```python
from build123d import *

# Parameters (mm, degrees)
SKETCH2_R           = 1.3
CUT_EXTRUDE1_DEPTH  = 15
BOSS_EXTRUDE1_START = 6
SKETCH3_R           = 2
SKETCH3_R_2         = 1.3
BOSS_EXTRUDE1_DEPTH = 6


with BuildPart() as part:
    # Sketch1 → Revolve2 (revolve)
    with BuildSketch(Plane.XY):
        with BuildLine():
            Line((-2.5, 0), (2.5, 0))
            ThreePointArc((2.5, 0), (0, -2.5), (-2.5, 0))
        make_face()
    revolve(axis=Axis((4.664316952, 0, 0), (-1, 0, 0)))

    # Sketch2 → Cut-Extrude1 (cut, symmetric)
    with BuildSketch(Plane(origin=(0, 0, 0), x_dir=(1, 0, 0), z_dir=(0, 1, 0))):
        with Locations(Location((0, 0, 0), (0, 0, 90))):
            Circle(SKETCH2_R)
    extrude(amount=CUT_EXTRUDE1_DEPTH, both=True, mode=Mode.SUBTRACT)

    # Sketch3 → Boss-Extrude1 (add)
    with BuildSketch(Plane(origin=(0, 0, 0), x_dir=(1, 0, 0), z_dir=(0, 1, 0)).offset(BOSS_EXTRUDE1_START)):
        with Locations(Location((0, 0, 0), (0, 0, 270))):
            Circle(SKETCH3_R)
        with Locations(Location((0, 0, 0), (0, 0, 270))):
            Circle(SKETCH3_R_2, mode=Mode.SUBTRACT)
    extrude(amount=-BOSS_EXTRUDE1_DEPTH)


solid = part.part
```
Could you check a few things on this model? Use its own coordinates, in mm. Coordinates: 2 decimals unless noted, no trailing zeros. Order: outer loops, then holes, each group sorted by start corner. A loop starts at its lowest first (then second) coordinate and runs counter-clockwise, first axis right, second up. Notation, with made-up numbers: M 1,78 L 21,78 A25 ccw 21,107 Z; hole C 77,-6 d7. An arc over 180 degrees is marked long. Use a Markdown table: item, result. Add a question column.
Q1. I want a section at C-C on y = 3.25. List the corners of the cut face in (x, z) for me.
Q2. I want a section at D-D on y = 1.25. List the corners of the cut face in (x, z) for me, then the cut area to 3 significant figures.
Q3. I'm going to push flat-ended pins straight in: pin 1 (1 mm diameter, centred on x = 2, y = 4, fed in from -Z); pin 2 (1.6 mm diameter, centred on x = 0, z = 0, fed in from -Y); pin 3 (3 mm diameter, centred on x = 0.5, y = 1.5, fed in from +Z). Where does each tip first touch, or does it pass through?
Q4. If I drill on L1, parallel to Z at x = -0.35, y = 4; L2, parallel to Z at x = 0.8, y = 4.25; L3, parallel to X at y = 4.5, z = 1.05, over which ranges is the centre line in solid material (lowest first)?
Q5. I want a section at A-A on x = 0. List the corners of the cut face in (y, z) for me.
Q6. I want a section at B-B on z = 0. List the corners of the cut face in (x, y) for me, then the cut area to 3 significant figures.
Checked values:
| question | item | result |
|---|---|---|
| 1 | outline | C 0,0 d4; hole C 0,0 d2.6 |
| 2 | outline | C 0,0 d4.33; hole C 0,0 d2.6 |
| 2 | area | 9.42 mm² |
| 3 | pin 1 | z = -1.32 |
| 3 | pin 2 | through |
| 3 | pin 3 | z = 2.5 |
| 4 | L1 | -1.97 to -1.25, 1.25 to 1.97 |
| 4 | L2 | -1.83 to -1.02, 1.02 to 1.83 |
| 4 | L3 | -1.7 to -0.77, 0.77 to 1.7 |
| 5 | outline | M -2.14,-1.3 A2.5 ccw 1.5,-2 L 6,-2 L 6,-1.3 Z; M -2.14,1.3 L 6,1.3 L 6,2 L 1.5,2 A2.5 ccw Z |
| 6 | outline | M -2,1.5 A2.5 ccw -1.3,-2.14 L -1.3,6 L -2,6 Z; M 1.3,-2.14 A2.5 ccw 2,1.5 L 2,6 L 1.3,6 Z |
| 6 | area | 13.0 mm² |
